Drawing for the job (mm, zero at the part's lowest x, y, z). A direction names the side the tool comes from. Give positions to 0.01 mm unless a question says otherwise; leave off trailing zeros. Order: outer loops, then holes, each group sorted by start corner. A loop starts at its lowest first (then second) coordinate and runs counter-clockwise, first axis right, second up. Notation, with made-up numbers: M 15,-6.75 L 48,-6.75 A28 cw 48,16.25 Z; hole C 6.5,77 d6. An arc over 180 degrees is marked long. One line per item, written item: value.
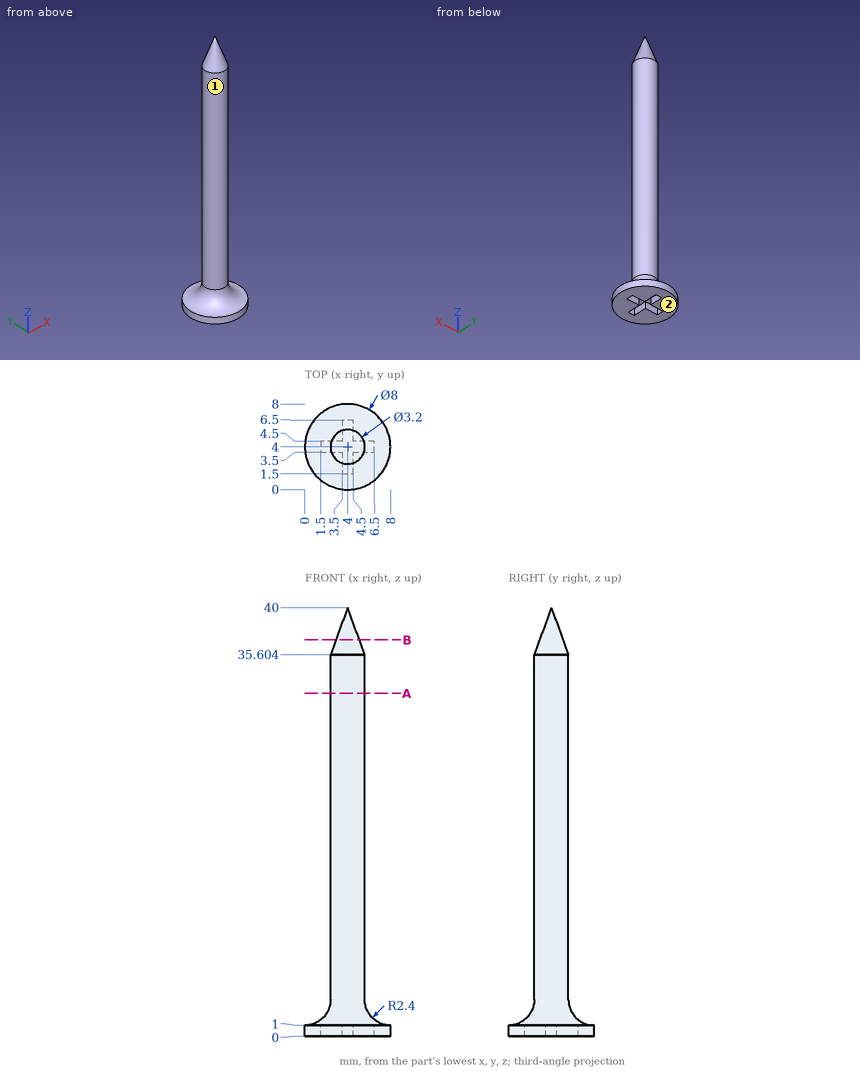
1) Pin check, flat tips, straight feed: pin 1 (0.8 mm diameter, centred on x = 2.5, z = 0.5, fed in from -Y); pin 2 (0.5 mm diameter, centred on x = 5, z = 0.5, fed in from +Y); pin 3 (1.5 mm diameter, centred on x = 3, z = 13.5, fed in from +Y). Stop position of each tip, or through.
Check values:
pin 1: y = 0.15
pin 2: y = 7.93
pin 3: y = 5.58
2) Tool access for the marked faces 1 and 2: list every direction of +Z, -Z, +X, -X, +Y, -Y with a clear straight run to the whole face (end or side of a thin tool).
Check values:
face 1: +Z
face 2: -Z, +X, -X, +Y, -Y
3) Saw through at B-B, the plane z = 37. Write the cut outline in (x, y), then the cut area to 3 significant figures.
Check values:
outline: C 4,4 d2.18
area: 3.75 mm^2
4) Drill centre lines: probe 1 along Y at (x, z) = (4, 28.5); probe 2 along X at (y, z) = (3.25, 7); probe 3 along Z at (x, y) = (2, 4). Where is each one in solid material? Low to high. Write a range as from..to.
Check values:
probe 1: 2.4..5.6
probe 2: 2.59..5.41
probe 3: 1..2.07
5) Saw through at A-A, the plane z = 32. Write the cut outline in (x, y), then the cut area to 3 significant figures.
Check values:
outline: C 4,4 d3.2
area: 8.04 mm^2
